The model under review builds one solid part; all positions refer to its coordinate system, in mm. A direction names the side the tool comes from. Coordinates: 2 decimals unless noted, no trailing zeros. Loops run counter-clockwise (first coordinate to the right, second up) from the corner with the lowest first, then second, coordinate; pieces in that order, holes last. Notation, with made-up numbers: (-39.75, -31) - (-26.75, -31) arc R10 ccw to (-26.75, -16) - close; hole circle Ø11 at (71.5, 88). An arc over 180 degrees is marked (long way). Answer in a Markdown table with one row per item. Add a question column.
(1) We need section B-B on x = -1. Write out the cut boundary in (y, z), plus the area to 3 significant figures.
(2) For line 1 along Z through (x, y) = (0.25, 5.75); line 2 along Z through (x, y) = (-2, 9.5); line 3 along X through (y, z) = (8, -3), list the stretches that pass through material, from the lowest coordinate up.
(3) We need section C-C on y = 6.75. Write out the cut boundary in (x, z), plus the area to 3 significant figures.
(4) Machinability: for faces 4 (the flat face through (0, 5, 3.5)), 5 (the flat face through (0, 0, 4)), which of the approach directions +Z, -Z, +X, -X, +Y, -Y give a long, thin tool a straight path to every point of the face, cutting with its end or side? Answer none if there is none.
(5) Mouldability with a two-part tool opening along Z and no side actions: class faces 1 (the cylindrical face through (14.985, 4.93, -0.66)), 2 (the cylindrical face through (4.95, 4.93, -0.05)), 3 (the flat face through (0, 10, 4)) as +Z half, -Z half, draft (parallel to the pull), parting line (faces both ways), or undercut.
(6) For P1, Ø1.5, axis at y = 6, z = -10.5, coming from the -X side; P2, Ø1.5, axis at y = 5, z = -9.5, coming from the +X side; P3, Ø4, axis at y = 7.5, z = 10, coming from the +X side, all flat-tipped, find the tip position at first contact; note any pin that passes through.
(7) We need section A-A on z = 0. Write out the cut boundary in (x, y), plus the area to 3 significant figures.
(8) We need section D-D on z = -6. Write out the cut boundary in (x, y).
Autodesk Inventor part; units mm, degrees
ref_plane "YZ Plane" through (0, 0, 0) normal (1, 0, 0) x (0, 1, 0)
ref_plane "XZ Plane" through (0, 0, 0) normal (0, 1, 0) x (-1, 0, 0)
ref_plane "XY Plane" through (0, 0, 0) normal (0, 0, 1) x (1, 0, 0)
sketch "Sketch1" plane through (0, 0, 0) normal (0, 1, 0) x (-1, 0, 0)
  circle A0 centre (0, 0) radius 15
  dimension "d0" = 30
extrude "Extrusion1" add sketch "Sketch1" along normal blind 10
sketch "Sketch2" plane through (0, 0, 0) normal (0, -1, 0) x (1, 0, 0)
  line L0 (-3.5, 3.5) -> (3.5, 3.5)
  line L1 (3.5, 3.5) -> (3.5, -3.5)
  line L2 (3.5, -3.5) -> (-3.5, -3.5)
  line L3 (-3.5, -3.5) -> (-3.5, 3.5)
  circle A0 centre (0, 0) radius 4.9497
  dimension "d3" = 7
  dimension "d4" = 7
  dimension "d5" = 3.5
  dimension "d6" = 3.5
extrude "Extrusion2" cut sketch "Sketch2" against normal blind 12.7 contours L0 L1 L2 L3 | L3 A0 | A0 L1
properties part number "generic-launcher-blank"
Outcome:
| question | item | result |
|---|---|---|
| 1 | outline | (0, -14.97) - (10, -14.97) - (10, -3.5) - (0, -3.5) - close; (0, 3.5) - (10, 3.5) - (10, 14.97) - (0, 14.97) - close |
| 1 | area | 229 mm² |
| 2 | line 1 | -15 to -3.5, 3.5 to 15 |
| 2 | line 2 | -14.87 to -3.5, 3.5 to 14.87 |
| 2 | line 3 | -14.7 to -3.94, 3.94 to 14.7 |
| 3 | outline | circle Ø30 at (0, 0); hole (-3.5, -3.5) - (3.5, -3.5) arc R4.95 ccw to (3.5, 3.5) - (-3.5, 3.5) arc R4.95 ccw to start |
| 3 | area | 644 mm² |
| 4 | face 4 | +Y, -Y |
| 4 | face 5 | +Z, -Z, +X, -X, -Y |
| 5 | face 1 | parting line |
| 5 | face 2 | undercut |
| 5 | face 3 | draft |
| 6 | P1 | x = -11.4 |
| 6 | P2 | x = 12.18 |
| 6 | P3 | x = 12.69 |
| 7 | outline | (-15, 0) - (-4.95, 0) - (-4.95, 10) - (-15, 10) - close; (4.95, 0) - (15, 0) - (15, 10) - (4.95, 10) - close |
| 7 | area | 201 mm² |
| 8 | outline | (-13.75, 0) - (13.75, 0) - (13.75, 10) - (-13.75, 10) - close |
